Part model, mm, in its own coordinate system. Round coordinates to 2 decimals unless told otherwise and drop trailing zeros. Write each loop counter-clockwise with the first axis right and the second up, starting at its lowest first coordinate (ties: lowest second). Pieces come first, ordered by that corner, then holes. Notation, with made-up numbers: M 15,49 L 71,49 A14 ccw 71,54 Z; hole C 2,43.5 d3. An arc over 180 degrees is marked long. Use a Markdown table: item, result. Add a question column.
1) Slice it at B-B on z = 0. Write the cut outline in (x, y) (1 decimal), plus the area to 3 significant figures.
2) Wall check: probe 1 along X at (y, z) = (1.65, 0); probe 2 along Z at (x, y) = (-31, 1.25); probe 3 along Z at (x, y) = (36.5, 0.75). Give the ranges that are in metal, low to high.
3) Slice it at A-A on x = 0. Write the cut outline in (y, z) (3 decimals), plus the area to 3 significant figures.
4) Drop flat-ended pins along their axis: P1, Ø5.5, axis at x = 85.725, z = 0, coming from the -Y side; P2, Ø4.5, axis at x = 42.86, z = 74.24, coming from the +Y side. Give the stop position or say it passes through.
5) Slice it at D-D on x = -28. Write the cut outline in (y, z) (3 decimals), plus the area to 3 significant figures.
6) Slice it at C-C on y = 1.1. Write the cut outline in (x, z) (1 decimal), plus the area to 3 significant figures.
7) Two-plate mould, pull along X, no slides. Class faces 1 (the face through (-40.83, 1.57, -72.94)), 2 (the face through (-46, 3.175, -24)), 3 (the face through (88.12, 1.57, -0.31)): released by +X, released by -X, zero draft, split by the parting line, or undercut.
```python
from build123d import *

# Parameters (mm, degrees)
SKETCH1_W           = 200.025
SKETCH1_H           = 203.2
SKETCH1_R           = 2.413
BOSS_EXTRUDE1_DEPTH = 3.175
SKETCH3_R           = 48.26
CUT_EXTRUDE1_DEPTH  = 143.601335131


with BuildPart() as part:
    # Sketch1 → Boss-Extrude1 (new body)
    with BuildSketch(Plane(origin=(0, 0, 0), x_dir=(1, 0, 0), z_dir=(0, 1, 0))):
        Rectangle(SKETCH1_W, SKETCH1_H)
        with Locations(Location((42.8625, 74.240027739, 0), (0, 0, 270))):
            Circle(SKETCH1_R, mode=Mode.SUBTRACT)
        with Locations(Location((85.725, 0, 0), (0, 0, 270))):
            Circle(SKETCH1_R, mode=Mode.SUBTRACT)
        with Locations(Location((42.8625, -74.240027739, 0), (0, 0, 270))):
            Circle(SKETCH1_R, mode=Mode.SUBTRACT)
        with Locations(Location((-42.8625, -74.240027739, 0), (0, 0, 270))):
            Circle(SKETCH1_R, mode=Mode.SUBTRACT)
        with Locations(Location((-85.725, 0, 0), (0, 0, 270))):
            Circle(SKETCH1_R, mode=Mode.SUBTRACT)
        with Locations(Location((-42.8625, 74.240027739, 0), (0, 0, 270))):
            Circle(SKETCH1_R, mode=Mode.SUBTRACT)
    extrude(amount=BOSS_EXTRUDE1_DEPTH)

    # Sketch3 → Cut-Extrude1 (cut, through all)
    with BuildSketch(Plane(origin=(0, 3.175, 0), x_dir=(1, 0, 0), z_dir=(0, 1, 0))):
        with Locations(Location((0, 0, 0), (0, 0, 270))):
            Circle(SKETCH3_R)
    extrude(amount=-CUT_EXTRUDE1_DEPTH, mode=Mode.SUBTRACT)


solid = part.part
```
Entries:
| question | item | result |
|---|---|---|
| 1 | outline | M -100,0 L -88.1,0 L -88.1,3.2 L -100,3.2 Z; M -83.3,0 L -48.3,0 L -48.3,3.2 L -83.3,3.2 Z; M 48.3,0 L 83.3,0 L 83.3,3.2 L 48.3,3.2 Z; M 88.1,0 L 100,0 L 100,3.2 L 88.1,3.2 Z |
| 1 | area | 298 mm^2 |
| 2 | probe 1 | x = -100.01 to -88.14, -83.31 to -48.26, 48.26 to 83.31, 88.14 to 100.01 |
| 2 | probe 2 | z = -101.6 to -36.99, 36.99 to 101.6 |
| 2 | probe 3 | z = -101.6 to -31.57, 31.57 to 101.6 |
| 3 | outline | M 0,-101.6 L 3.175,-101.6 L 3.175,-48.26 L 0,-48.26 Z; M 0,48.26 L 3.175,48.26 L 3.175,101.6 L 0,101.6 Z |
| 3 | area | 339 mm^2 |
| 4 | P1 | stops at y = 0 |
| 4 | P2 | passes through |
| 5 | outline | M 0,-101.6 L 3.175,-101.6 L 3.175,-39.307 L 0,-39.307 Z; M 0,39.307 L 3.175,39.307 L 3.175,101.6 L 0,101.6 Z |
| 5 | area | 396 mm^2 |
| 6 | outline | M -100,-101.6 L 100,-101.6 L 100,101.6 L -100,101.6 Z; hole C -85.7,0 d4.8; hole C 0,0 d96.5; hole C -42.9,-74.2 d4.8; hole C -42.9,74.2 d4.8; hole C 42.9,-74.2 d4.8; hole C 42.9,74.2 d4.8; hole C 85.7,0 d4.8 |
| 6 | area | 33,200 mm^2 |
| 7 | face 1 | undercut |
| 7 | face 2 | zero draft |
| 7 | face 3 | undercut |
